```python
from build123d import *

# Parameters (mm, degrees)
SKETCH_W        = 150
SKETCH_H        = 200
SKETCH_R        = 1.75
PAD_DEPTH       = 3
SKETCH001_W     = 150
SKETCH001_H     = 200
PAD001_DEPTH    = 7
SKETCH005_W     = 13
SKETCH005_H     = 13
PAD002_DEPTH    = 3
SKETCH002_R     = 1.75
POCKET_DEPTH    = 5
SKETCH003_R     = 1.75
POCKET001_DEPTH = 5
SKETCH004_R     = 1.75
POCKET002_DEPTH = 14


with BuildPart() as part:
    # Sketch → Pad (new body)
    with BuildSketch(Plane.XY):
        with Locations((-75, 100)):
            Rectangle(SKETCH_W, SKETCH_H)
        with Locations((-140, 40)):
            Circle(SKETCH_R, mode=Mode.SUBTRACT)
        with Locations((-130, 40)):
            Circle(SKETCH_R, mode=Mode.SUBTRACT)
        with Locations((-120, 40)):
            Circle(SKETCH_R, mode=Mode.SUBTRACT)
        with Locations((-110, 40)):
            Circle(SKETCH_R, mode=Mode.SUBTRACT)
        with Locations((-100, 40)):
            Circle(SKETCH_R, mode=Mode.SUBTRACT)
        with Locations((-90, 40)):
            Circle(SKETCH_R, mode=Mode.SUBTRACT)
        with Locations((-80, 40)):
            Circle(SKETCH_R, mode=Mode.SUBTRACT)
        with Locations((-70, 40)):
            Circle(SKETCH_R, mode=Mode.SUBTRACT)
        with Locations((-60, 40)):
            Circle(SKETCH_R, mode=Mode.SUBTRACT)
        with Locations((-50, 40)):
            Circle(SKETCH_R, mode=Mode.SUBTRACT)
        with Locations((-40, 40)):
            Circle(SKETCH_R, mode=Mode.SUBTRACT)
        with Locations((-30, 40)):
            Circle(SKETCH_R, mode=Mode.SUBTRACT)
        with Locations((-20, 40)):
            Circle(SKETCH_R, mode=Mode.SUBTRACT)
        with Locations((-10, 40)):
            Circle(SKETCH_R, mode=Mode.SUBTRACT)
        with Locations((-140, 50)):
            Circle(SKETCH_R, mode=Mode.SUBTRACT)
        with Locations((-130, 50)):
            Circle(SKETCH_R, mode=Mode.SUBTRACT)
        with Locations((-120, 50)):
            Circle(SKETCH_R, mode=Mode.SUBTRACT)
        with Locations((-110, 50)):
            Circle(SKETCH_R, mode=Mode.SUBTRACT)
        with Locations((-100, 50)):
            Circle(SKETCH_R, mode=Mode.SUBTRACT)
        with Locations((-90, 50)):
            Circle(SKETCH_R, mode=Mode.SUBTRACT)
        with Locations((-80, 50)):
            Circle(SKETCH_R, mode=Mode.SUBTRACT)
        with Locations((-70, 50)):
            Circle(SKETCH_R, mode=Mode.SUBTRACT)
        with Locations((-60, 50)):
            Circle(SKETCH_R, mode=Mode.SUBTRACT)
        with Locations((-50, 50)):
            Circle(SKETCH_R, mode=Mode.SUBTRACT)
        with Locations((-40, 50)):
            Circle(SKETCH_R, mode=Mode.SUBTRACT)
        with Locations((-30, 50)):
            Circle(SKETCH_R, mode=Mode.SUBTRACT)
        with Locations((-20, 50)):
            Circle(SKETCH_R, mode=Mode.SUBTRACT)
        with Locations((-10, 50)):
            Circle(SKETCH_R, mode=Mode.SUBTRACT)
        with Locations((-140, 140)):
            Circle(SKETCH_R, mode=Mode.SUBTRACT)
        with Locations((-130, 140)):
            Circle(SKETCH_R, mode=Mode.SUBTRACT)
        with Locations((-120, 140)):
            Circle(SKETCH_R, mode=Mode.SUBTRACT)
        with Locations((-110, 140)):
            Circle(SKETCH_R, mode=Mode.SUBTRACT)
        with Locations((-100, 140)):
            Circle(SKETCH_R, mode=Mode.SUBTRACT)
        with Locations((-90, 140)):
            Circle(SKETCH_R, mode=Mode.SUBTRACT)
        with Locations((-80, 140)):
            Circle(SKETCH_R, mode=Mode.SUBTRACT)
        with Locations((-70, 140)):
            Circle(SKETCH_R, mode=Mode.SUBTRACT)
        with Locations((-60, 140)):
            Circle(SKETCH_R, mode=Mode.SUBTRACT)
        with Locations((-50, 140)):
            Circle(SKETCH_R, mode=Mode.SUBTRACT)
        with Locations((-40, 140)):
            Circle(SKETCH_R, mode=Mode.SUBTRACT)
        with Locations((-30, 140)):
            Circle(SKETCH_R, mode=Mode.SUBTRACT)
        with Locations((-20, 140)):
            Circle(SKETCH_R, mode=Mode.SUBTRACT)
        with Locations((-10, 140)):
            Circle(SKETCH_R, mode=Mode.SUBTRACT)
        with Locations((-140, 150)):
            Circle(SKETCH_R, mode=Mode.SUBTRACT)
        with Locations((-130, 150)):
            Circle(SKETCH_R, mode=Mode.SUBTRACT)
        with Locations((-120, 150)):
            Circle(SKETCH_R, mode=Mode.SUBTRACT)
        with Locations((-110, 150)):
            Circle(SKETCH_R, mode=Mode.SUBTRACT)
        with Locations((-100, 150)):
            Circle(SKETCH_R, mode=Mode.SUBTRACT)
        with Locations((-90, 150)):
            Circle(SKETCH_R, mode=Mode.SUBTRACT)
        with Locations((-80, 150)):
            Circle(SKETCH_R, mode=Mode.SUBTRACT)
        with Locations((-70, 150)):
            Circle(SKETCH_R, mode=Mode.SUBTRACT)
        with Locations((-60, 150)):
            Circle(SKETCH_R, mode=Mode.SUBTRACT)
        with Locations((-50, 150)):
            Circle(SKETCH_R, mode=Mode.SUBTRACT)
        with Locations((-40, 150)):
            Circle(SKETCH_R, mode=Mode.SUBTRACT)
        with Locations((-30, 150)):
            Circle(SKETCH_R, mode=Mode.SUBTRACT)
        with Locations((-20, 150)):
            Circle(SKETCH_R, mode=Mode.SUBTRACT)
        with Locations((-10, 150)):
            Circle(SKETCH_R, mode=Mode.SUBTRACT)
        with Locations((-125, 193.5)):
            Circle(SKETCH_R, mode=Mode.SUBTRACT)
        with Locations((-125, 6.5)):
            Circle(SKETCH_R, mode=Mode.SUBTRACT)
        with Locations((-25, 6.5)):
            Circle(SKETCH_R, mode=Mode.SUBTRACT)
        with Locations((-75, 6.5)):
            Circle(SKETCH_R, mode=Mode.SUBTRACT)
        with Locations((-25, 193.5)):
            Circle(SKETCH_R, mode=Mode.SUBTRACT)
        with Locations((-75, 193.5)):
            Circle(SKETCH_R, mode=Mode.SUBTRACT)
    extrude(amount=PAD_DEPTH)

    # Sketch001 (on DatumPlane) → Pad001 (join)
    with BuildSketch(Plane.XY.offset(3)):
        with Locations((-75, 100)):
            Rectangle(SKETCH001_W, SKETCH001_H)
        Polygon((-147, 197), (-13, 197), (-13, 187), (-3, 187), (-3, 13), (-13, 13), (-13, 3), (-147, 3), align=None, mode=Mode.SUBTRACT)
    extrude(amount=PAD001_DEPTH)

    # Sketch005 (on DatumPlane) → Pad002 (join)
    with BuildSketch(Plane.XY.offset(10)):
        with Locations((-6.5, 193.5)):
            Rectangle(SKETCH005_W, SKETCH005_H)
        with Locations((-6.5, 6.5)):
            Rectangle(SKETCH005_W, SKETCH005_H)
    extrude(amount=PAD002_DEPTH)

    # Sketch002 → Pocket (cut)
    with BuildSketch(Plane.YZ):
        with Locations((100, 6.5)):
            Circle(SKETCH002_R)
        with Locations((22, 6.5)):
            Circle(SKETCH002_R)
        with Locations((178, 6.5)):
            Circle(SKETCH002_R)
    extrude(amount=-POCKET_DEPTH, mode=Mode.SUBTRACT)

    # Sketch003 → Pocket001 (cut)
    with BuildSketch(Plane.YZ.offset(-150)):
        with Locations((100, 6.5)):
            Circle(SKETCH003_R)
        with Locations((22, 6.5)):
            Circle(SKETCH003_R)
        with Locations((178, 6.5)):
            Circle(SKETCH003_R)
    extrude(amount=POCKET001_DEPTH, mode=Mode.SUBTRACT)

    # Sketch004 → Pocket002 (cut)
    with BuildSketch(Plane.XZ):
        with Locations((-6.5, 6.5)):
            Circle(SKETCH004_R)
    extrude(amount=-POCKET002_DEPTH, mode=Mode.SUBTRACT)


solid = part.part
```
Geometry: final body of the model. Coordinates: model frame, mm. A direction names the side the tool comes from. Give positions to 0.01 mm unless a question says otherwise; leave off trailing zeros. Order: outer loops, then holes, each group sorted by start corner. A loop starts at its lowest first (then second) coordinate and runs counter-clockwise, first axis right, second up. Notation, with made-up numbers: (49, 24) -> (60, 24) arc R14 cw to (60, 50) -> close; hole circle Ø10 at (61.25, 86.25). An arc over 180 degrees is marked (long way). Write each question's results on one line, items separated by ' | '. Start each with the question number.
1) Draft query along X for faces 3 (the flat face through (-148, 100, 10)), 4 (the flat face through (-79, 3, 6)), 5 (the flat face through (-147, 98.6, 8)), 6 (the flat face through (-150, 98.6, 4.9)). Return one class per face: pulls with the +X half, pulls with the -X half, needs draft (parallel to the pull), parting line crosses it, or undercut.
2) Line query: line 1 (Y direction, x = -75, z = 0.85); line 2 (Y direction, x = -50, z = 1.4); line 3 (Y direction, x = -148.1, z = 6.5). Output: solid intervals per line, ascending. Write a range as from..to.
3) Set-up query: faces 1 (the flat face through (-81, 197, 6)), 2 (the flat face through (-76, 0, 5)). Return all of +Z, -Z, +X, -X, +Y, -Y with unobstructed straight access to the full face (end or side cutting, diameter ignored); none if empty.
4) Section A-A (x = -115.5). Return loops of the section in (y, z), then the cut area to 3 significant figures.
5) First-contact query: pin 1 (4.5 mm diameter, centred on x = -140, y = 40, fed in from +Z); pin 2 (3 mm diameter, centred on x = -50, y = 50, fed in from -Z). Flat tips, straight axial feed; report the tip coordinate or a pass-through.
6) Section B-B (y = 183). Return loops of the section in (x, z), then the cut area to 3 significant figures.
Calculated:
1) face 3: needs draft | face 4: undercut | face 5: undercut | face 6: pulls with the -X half
2) line 1: 0..4.75, 8.25..191.75, 195.25..200 | line 2: 0..38.25, 41.75..48.25, 51.75..138.25, 141.75..148.25, 151.75..200 | line 3: 0..20.25, 23.75..98.25, 101.75..176.25, 179.75..200
3) face 1: +Z | face 2: +Z, -Z, +X, -X, -Y
4) outline: (0, 0) -> (200, 0) -> (200, 10) -> (197, 10) -> (197, 3) -> (3, 3) -> (3, 10) -> (0, 10) -> close | area: 642 mm2
5) pin 1: z = 3 | pin 2: through
6) outline: (-150, 0) -> (0, 0) -> (0, 10) -> (-3, 10) -> (-3, 3) -> (-147, 3) -> (-147, 10) -> (-150, 10) -> close | area: 492 mm2
